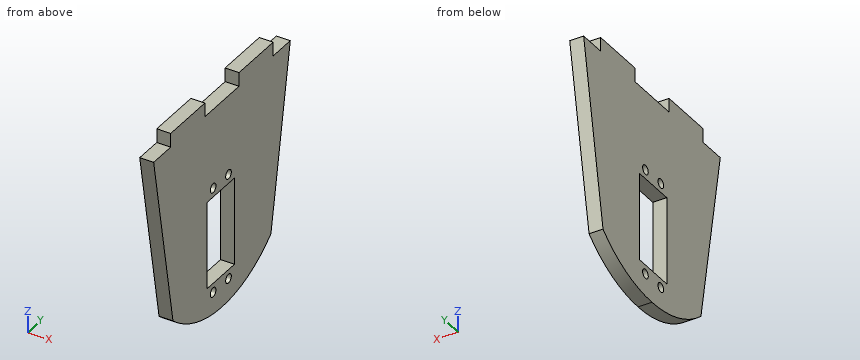
from build123d import *

# Parameters (mm, degrees)
F1_DEPTH = 6.35
F2_W     = 12.7
F2_H     = 6.35
F3_DEPTH = 25.4
F4_W     = 20.32
F4_H     = 40.005
F4_R     = 2.0955
F5_DEPTH = 25.4


# Not quite as in the source:
# - a feature names something its author has since deleted; it is built from what else it names


with BuildPart() as f1:
    # F0 (on Right) → F1 (new body)
    with BuildSketch(Plane.YZ):
        with BuildLine():
            Line((50.8, 0), (0, 0))
            Line((0, 0), (0, -6.35))
            Line((0, -6.35), (14.3783799252, -87.8938446653))
            ThreePointArc((14.3783799252, -87.8938446653), (31.3423979963, -98.0600456848), (50.8, -101.6))
            Line((50.8, -101.6), (50.8, 0))
        make_face()
        with BuildLine():
            Line((101.6, 0), (50.8, 0))
            Line((50.8, 0), (50.8, -101.6))
            ThreePointArc((50.8, -101.6), (70.2576020037, -98.0600456848), (87.2216200748, -87.8938446653))
            Line((87.2216200748, -87.8938446653), (101.6, -6.35))
            Line((101.6, -6.35), (101.6, 0))
        make_face()
    extrude(amount=F1_DEPTH)

    # F2 (on face) → F3 (cut)
    with BuildSketch(Plane.YZ.offset(6.35)):
        with Locations((95.25, -3.175)):
            Rectangle(F2_W, F2_H)
        with Locations((44.45, -3.175)):
            Rectangle(F2_W, F2_H)
        with Locations((6.35, -3.175)):
            Rectangle(F2_W, F2_H)
        with Locations((57.15, -3.175)):
            Rectangle(F2_W, F2_H)
    extrude(amount=-F3_DEPTH, mode=Mode.SUBTRACT)

    # F4 (on face) → F5 (cut)
    with BuildSketch(Plane.YZ.offset(6.35)):
        with Locations((49.9361574873, -66.9925)):
            Rectangle(F4_W, F4_H)
        with Locations((44.2211574873, -42.8625)):
            Circle(F4_R)
        with Locations((55.6511574873, -42.8625)):
            Circle(F4_R)
        with Locations((55.6511574873, -91.1225)):
            Circle(F4_R)
        with Locations((44.2211574873, -91.1225)):
            Circle(F4_R)
    extrude(amount=-F5_DEPTH, mode=Mode.SUBTRACT)


solid = f1.part
For this review, take the finished solid that the model builds, in its own axes (mm). Coordinates: 2 decimals unless noted, no trailing zeros. Write each loop counter-clockwise with the first axis right and the second up, starting at its lowest first coordinate (ties: lowest second). Pieces come first, ordered by that corner, then holes. Notation, with made-up numbers: (-27, -33.5) -> (-13, -33.5) arc R31 cw to (-13, -9.5) -> close; hole circle Ø5 at (60, 5.25). An arc over 180 degrees is marked (long way). Write each question's results on one line, items separated by ' | '. Start each with the question number.
1) Insertion check: pin 1 (1 mm diameter, centred on x = 4.5, y = 65.5, fed in from -Z); pin 2 (3 mm diameter, centred on x = 4, z = -3.5, fed in from -Y); pin 3 (3 mm diameter, centred on x = 1, y = 15.5, fed in from -Z). Each pin has a flat end and moves straight along its axis. Give the tip position at first contact, or say it passes through.
2) Consider section B-B (x = 4.75). Give the number of separate pieces and of enclosed holes in the cut face, plus the area to 3 significant figures.
3) Wall thickness on L1, parallel to Z at x = 4, y = 54 (3 decimals); L2, parallel to Y at x = 2, z = -6.5; L3, parallel to Z at x = 4.25, y = 47.5 (3 decimals): over which ranges is each line inside the solid? List them lowest first. Write a range as [from, to].
4) Consider section C-C (y = 25.5). Write out the cut boundary in (x, z).
5) Consider section A-A (y = 48). Write out the cut boundary in (x, z) (3 decimals), plus the area to 3 significant figures.
Geometry says:
1) pin 1: z = -99.74 | pin 2: y = 12.7 | pin 3: z = -90.05
2) separate pieces: 1 | enclosed holes: 5 | area: 7,250 mm^2
3) L1: [-101.507, -92.413], [-89.832, -86.995], [-46.99, -44.153], [-41.572, -6.35] | L2: [0.03, 101.57] | L3: [-101.501, -86.995], [-46.99, -6.35]
4) outline: (0, -95.47) -> (6.35, -95.47) -> (6.35, 0) -> (0, 0) -> close
5) outline: (0, -101.529) -> (6.35, -101.529) -> (6.35, -86.995) -> (0, -86.995) -> close; (0, -46.99) -> (6.35, -46.99) -> (6.35, -6.35) -> (0, -6.35) -> close | area: 350 mm^2
